Work out the finished part from the listing and answer in its coordinate system (mm). A direction names the side the tool comes from. Coordinates: 2 decimals unless noted, no trailing zeros. Order: outer loops, then holes, each group sorted by start corner. A loop starts at its lowest first (then second) coordinate and runs counter-clockwise, first axis right, second up. Notation, with made-up numbers: M -29,-13.75 L 8,-13.75 A18 cw 8,-4.75 Z; hole C 84,37.25 d4. An arc over 180 degrees is marked long. Use a Markdown table: item, result.
from build123d import *

# Parameters (mm, degrees)
SKETCH1_R           = 3.556
BOSS_EXTRUDE1_DEPTH = 76.2
SKETCH2_R           = 1.905
CUT_EXTRUDE1_DEPTH  = 6.604
BOSS_EXTRUDE2_DEPTH = 17.78
SKETCH4_W           = 6.858
SKETCH4_H           = 2.54
SKETCH4_W_2         = 2.54
SKETCH4_H_2         = 10.16
SKETCH4_H_3         = 18.288
BOSS_EXTRUDE3_DEPTH = 7.112
SKETCH5_R           = 1.905
CUT_EXTRUDE3_DEPTH  = 7.112
SKETCH6_R           = 1.905
CUT_EXTRUDE4_DEPTH  = 7.112
SKETCH8_W           = 0.508
SKETCH8_H           = 20.32
CUT_EXTRUDE5_DEPTH  = 17.78
SKETCH9_W           = 0.508
SKETCH9_H           = 2.54
CUT_EXTRUDE6_DEPTH  = 7.112
SKETCH10_W          = 0.508
SKETCH10_H          = 12.7
SKETCH10_H_2        = 23.368
CUT_EXTRUDE7_DEPTH  = 7.112
SKETCH11_W          = 57.041716114
SKETCH11_H          = 0.508
CUT_EXTRUDE8_DEPTH  = 17.78


with BuildPart() as part:
    # Sketch1 → Boss-Extrude1 (new body)
    with BuildSketch(Plane.XY):
        with BuildLine():
            Line((-44.45, 6.096), (44.45, 6.096))
            ThreePointArc((44.45, 6.096), (50.546, 0), (44.45, -6.096))
            Line((44.45, -6.096), (-44.45, -6.096))
            ThreePointArc((-44.45, -6.096), (-50.546, 0), (-44.45, 6.096))
        make_face()
        with Locations((-44.45, 0)):
            Circle(SKETCH1_R, mode=Mode.SUBTRACT)
        with Locations((44.45, 0)):
            Circle(SKETCH1_R, mode=Mode.SUBTRACT)
    extrude(amount=BOSS_EXTRUDE1_DEPTH)

    # Sketch2 → Cut-Extrude1 (cut)
    with BuildSketch(Plane.XZ.offset(6.096)):
        with Locations((-9.144, 69.215)):
            Circle(SKETCH2_R)
        with Locations((27.051, 60.833)):
            Circle(SKETCH2_R)
        with Locations((-28.956, 69.215)):
            Circle(SKETCH2_R)
        with Locations((-28.956, 6.985)):
            Circle(SKETCH2_R)
        with Locations((-9.144, 6.985)):
            Circle(SKETCH2_R)
        with Locations((11.049, 60.833)):
            Circle(SKETCH2_R)
        with Locations((11.049, 15.367)):
            Circle(SKETCH2_R)
        with Locations((27.051, 15.367)):
            Circle(SKETCH2_R)
    extrude(amount=-CUT_EXTRUDE1_DEPTH, mode=Mode.SUBTRACT)

    # Sketch3 → Boss-Extrude2 (add)
    with BuildSketch(Plane(origin=(0, 6.096, 0), x_dir=(1, 0, 0), z_dir=(0, 1, 0))):
        Polygon((-29.21, -10.16), (-29.21, -44.45), (29.21, -44.45), (29.21, -41.91), (-26.67, -41.91), (-26.67, -12.7), (26.307716114, -12.7), (26.307716114, -30.48), (28.847716114, -30.48), (28.847716114, -10.16), align=None)
    extrude(amount=BOSS_EXTRUDE2_DEPTH)

    # Sketch4 → Boss-Extrude3 (add)
    with BuildSketch(Plane(origin=(0, 6.096, 0), x_dir=(1, 0, 0), z_dir=(0, 1, 0))):
        with Locations((-32.639, -43.18)):
            Rectangle(SKETCH4_W, SKETCH4_H)
        with Locations((-34.798, -57.658)):
            Rectangle(SKETCH4_W_2, SKETCH4_H_2)
        Polygon((36.068, -62.738), (33.528, -62.738), (-33.528, -62.738), (-36.068, -62.738), (-36.068, -65.278), (36.068, -65.278), align=None)
        with Locations((34.798, -53.594)):
            Rectangle(SKETCH4_W_2, SKETCH4_H_3)
        with Locations((32.639, -43.18)):
            Rectangle(SKETCH4_W, SKETCH4_H)
    extrude(amount=BOSS_EXTRUDE3_DEPTH)

    # Sketch5 → Cut-Extrude3 (cut)
    with BuildSketch(Plane(origin=(0, 6.096, 0), x_dir=(1, 0, 0), z_dir=(0, 1, 0))):
        with Locations((36.068, -67.818)):
            Circle(SKETCH5_R)
        with Locations((32.911716114, -6.35)):
            Circle(SKETCH5_R)
    extrude(amount=-CUT_EXTRUDE3_DEPTH, mode=Mode.SUBTRACT)

    # Sketch6 → Cut-Extrude4 (cut)
    with BuildSketch(Plane(origin=(0, 6.096, 0), x_dir=(1, 0, 0), z_dir=(0, 1, 0))):
        with Locations((-33.274, -6.35)):
            Circle(SKETCH6_R)
        with Locations((-36.322, -67.818)):
            Circle(SKETCH6_R)
    extrude(amount=-CUT_EXTRUDE4_DEPTH, mode=Mode.SUBTRACT)

    # Sketch8 → Cut-Extrude5 (cut)
    with BuildSketch(Plane(origin=(0, 23.876, 0), x_dir=(1, 0, 0), z_dir=(0, 1, 0))):
        with Locations((28.593716114, -20.32)):
            Rectangle(SKETCH8_W, SKETCH8_H)
        Polygon((-28.702, -41.91), (-28.702, -10.16), (-29.21, -10.16), (-29.21, -41.825929555), align=None)
    extrude(amount=-CUT_EXTRUDE5_DEPTH, mode=Mode.SUBTRACT)

    # Sketch9 → Cut-Extrude6 (cut)
    with BuildSketch(Plane(origin=(0, 13.208, 0), x_dir=(1, 0, 0), z_dir=(0, 1, 0))):
        with Locations((-35.814, -43.18)):
            Rectangle(SKETCH9_W, SKETCH9_H)
    extrude(amount=-CUT_EXTRUDE6_DEPTH, mode=Mode.SUBTRACT)

    # Sketch10 → Cut-Extrude7 (cut)
    with BuildSketch(Plane(origin=(0, 13.208, 0), x_dir=(1, 0, 0), z_dir=(0, 1, 0))):
        with Locations((-35.814, -58.928)):
            Rectangle(SKETCH10_W, SKETCH10_H)
        with Locations((35.814, -53.594)):
            Rectangle(SKETCH10_W, SKETCH10_H_2)
    extrude(amount=-CUT_EXTRUDE7_DEPTH, mode=Mode.SUBTRACT)

    # Sketch11 → Cut-Extrude8 (cut)
    with BuildSketch(Plane(origin=(0, 23.876, 0), x_dir=(1, 0, 0), z_dir=(0, 1, 0))):
        with Locations((-0.181141943, -10.414)):
            Rectangle(SKETCH11_W, SKETCH11_H)
    extrude(amount=-CUT_EXTRUDE8_DEPTH, mode=Mode.SUBTRACT)


solid = part.part
1. Section A-A on z = 37.5 is taken. Determine the outline of the cut face in (x, y), then the cut area to 3 significant figures.
Answers below:
| item | result |
|---|---|
| outline | M -44.45,-6.1 L 44.45,-6.1 A6.1 ccw 44.45,6.1 L -26.67,6.1 L -26.67,23.88 L -28.7,23.88 L -28.7,6.1 L -44.45,6.1 A6.1 ccw Z; hole C -44.45,0 d7.11; hole C 44.45,0 d7.11 |
| area | 1,160 mm² |
2. For a pull along Z with two mould halves and no side action, classify faces 1 (the face through (-34.505, 2.59, 67.246)), 2 (the face through (-32, 13.208, 43)), 3 (the face through (10.636, -2.84, 58.973)), 4 (the face through (-32, 10, 41.91)) as +Z half, -Z half, draft (parallel to the pull), parting line (faces both ways), or undercut.
Answers below:
| item | result |
|---|---|
| face 1 | undercut |
| face 2 | draft |
| face 3 | undercut |
| face 4 | -Z half |
3. Flat-ended cylindrical pins translate along their axes: P1, Ø5.5, axis at x = 15, y = 11, coming from the +Z side; P2, Ø12, axis at y = 15.5, z = 15, coming from the -X side; P3, Ø14, axis at y = 14, z = 23, coming from the +X side. Find the tip coordinate at first contact, or state that the pin passes through.
Answers below:
| item | result |
|---|---|
| P1 | z = 65.28 |
| P2 | x = -28.7 |
| P3 | x = 28.34 |
4. Section D-D on z = 50.5 is taken. Determine the outline of the cut face in (x, y), then the cut area to 3 significant figures.
Answers below:
| item | result |
|---|---|
| outline | M -44.45,-6.1 L 44.45,-6.1 A6.1 ccw 44.45,6.1 L 35.56,6.1 L 35.56,13.21 L 33.53,13.21 L 33.53,6.1 L -44.45,6.1 A6.1 ccw Z; hole C -44.45,0 d7.11; hole C 44.45,0 d7.11 |
| area | 1,140 mm² |
5. Section C-C on y = 18 is taken. Determine the outline of the cut face in (x, z), then the cut area to 3 significant figures.
Answers below:
| item | result |
|---|---|
| outline | M -29.21,41.83 L -28.7,41.91 L -28.7,10.67 L 28.34,10.67 L 28.34,30.48 L 26.31,30.48 L 26.31,12.7 L -26.67,12.7 L -26.67,41.91 L 29.21,41.91 L 29.21,44.45 L -29.21,44.45 Z |
| area | 360 mm² |
6. Section B-B on x = -24 is taken. Determine the outline of the cut face in (y, z), then the cut area to 3 significant figures.
Answers below:
| item | result |
|---|---|
| outline | M -6.1,0 L 6.1,0 L 6.1,10.67 L 23.88,10.67 L 23.88,12.7 L 6.1,12.7 L 6.1,41.91 L 23.88,41.91 L 23.88,44.45 L 6.1,44.45 L 6.1,62.74 L 13.21,62.74 L 13.21,65.28 L 6.1,65.28 L 6.1,76.2 L -6.1,76.2 Z |
| area | 1,030 mm² |
7. For faces 5 (the face through (-29, 0.508, 7)), 6 (the face through (29.21, 18, 43)), 7 (the face through (0, 10, 62.738)), determine the directions among +Z, -Z, +X, -X, +Y, -Y from which every point of the face is accessible in a straight line to the end or side of a thin tool.
Answers below:
| item | result |
|---|---|
| face 5 | -Y |
| face 6 | +Z, -Z, +X, +Y |
| face 7 | +Y |
8. Find the intervals of material crossed by probe 1 along X at (y, z) = (-0.25, 26.5); probe 2 along Z at (x, y) = (2.5, 6.5); probe 3 along Z at (x, y) = (22, 21.25), in increasing order.
Answers below:
| item | result |
|---|---|
| probe 1 | -50.54 to -48, -40.9 to 40.9, 48 to 50.54 |
| probe 2 | 10.67 to 12.7, 41.91 to 44.45, 62.74 to 65.28 |
| probe 3 | 10.67 to 12.7, 41.91 to 44.45 |
